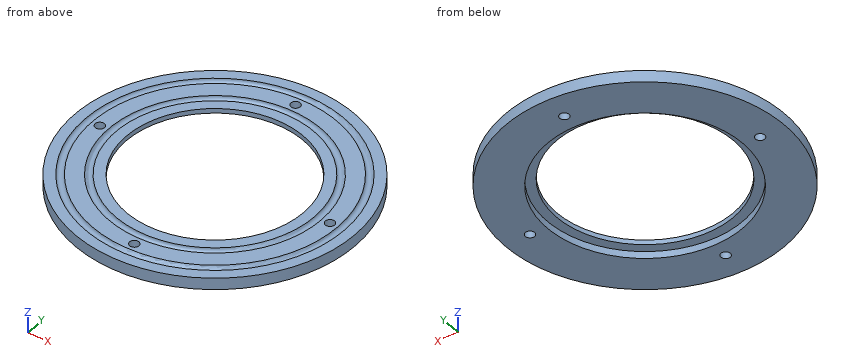
```python
from build123d import *

# Parameters (mm, degrees)
SKETCH4_R          = 2
CUT_EXTRUDE1_DEPTH = 10
SKETCH5_R          = 42
CUT_EXTRUDE2_DEPTH = 3


with BuildPart() as part:
    # Sketch3 → Revolve1 (revolve)
    with BuildSketch(Plane(origin=(0, 0, 0), x_dir=(1, 0, 0), z_dir=(0, 1, 0))):
        with BuildLine():
            Line((60, 0), (60, 5))
            Line((60, 5), (38, 5))
            Line((38, 5), (38, 0))
            Line((38, 0), (42.5, 0))
            ThreePointArc((42.5, 0), (44, 1.5), (45.5, 0))
            Line((45.5, 0), (52.5, 0))
            ThreePointArc((52.5, 0), (54, 1.5), (55.5, 0))
            Line((55.5, 0), (60, 0))
        make_face()
    revolve(axis=Axis((0, 0, 0), (0, 0, -1)))

    # Sketch4 → Cut-Extrude1 (cut)
    with BuildSketch(Plane.XY):
        with Locations((49, 0)):
            Circle(SKETCH4_R)
        with Locations((-49, 0)):
            Circle(SKETCH4_R)
        with Locations((0, 49)):
            Circle(SKETCH4_R)
        with Locations((0, -49)):
            Circle(SKETCH4_R)
    extrude(amount=-CUT_EXTRUDE1_DEPTH, mode=Mode.SUBTRACT)

    # Sketch5 → Cut-Extrude2 (cut)
    with BuildSketch(Plane(origin=(0, 0, -5), x_dir=(-1, 0, 0), z_dir=(0, 0, -1))):
        Circle(SKETCH5_R)
    extrude(amount=-CUT_EXTRUDE2_DEPTH, mode=Mode.SUBTRACT)


solid = part.part
```
Here's how the part is built. I have some questions about the finished solid (model axes, mm). Coordinates: 2 decimals unless noted, no trailing zeros. Loops run counter-clockwise (first coordinate to the right, second up) from the corner with the lowest first, then second, coordinate; pieces in that order, holes last. Notation, with made-up numbers: (66, 46.5) -> (71, 46.5) arc R10 cw to (71, 63.5) -> close; hole circle Ø7 at (-35, -12). An arc over 180 degrees is marked (long way). Return JSON: item names as keys, results as strings.
1) I need wall thicknesses on line 1 (Y direction, x = 0, z = -2.6); line 2 (Y direction, x = -24.5, z = -0.55); line 3 (Y direction, x = -1, z = -3.1). Which ranges of each line are inside material? Lowest first, please. Write a range as from..to.
Results below:
{"line 1": "-60..-51, -47..-42, 42..47, 51..60", "line 2": "-54.77..-49.68, -46.55..-38.22, -34.86..-29.05, 29.05..34.86, 38.22..46.55, 49.68..54.77", "line 3": "-59.99..-50.73, -47.27..-41.99, 41.99..47.27, 50.73..59.99"}
2) If we section it at C-C, the plane z = -3.35: Write out the boundary of the cut face in (x, y), then the cut area to 3 significant figures.
Results below:
{"outline": "circle Ø120 at (0, 0); hole circle Ø4 at (-49, 0); hole circle Ø84 at (0, 0); hole circle Ø4 at (0, -49); hole circle Ø4 at (0, 49); hole circle Ø4 at (49, 0)", "area": "5,720 mm²"}
3) If we section it at A-A, the plane x = 0: Write out the boundary of the cut face in (y, z), then the cut area to 3 significant figures.
Results below:
{"outline": "(-60, -5) -> (-51, -5) -> (-51, 0) -> (-52.5, 0) arc R1.5 cw to (-55.5, 0) -> (-60, 0) -> close; (-47, -5) -> (-42, -5) -> (-42, -2) -> (-38, -2) -> (-38, 0) -> (-42.5, 0) arc R1.5 cw to (-45.5, 0) -> (-47, 0) -> close; (38, -2) -> (42, -2) -> (42, -5) -> (47, -5) -> (47, 0) -> (45.5, 0) arc R1.5 cw to (42.5, 0) -> (38, 0) -> close; (51, -5) -> (60, -5) -> (60, 0) -> (55.5, 0) arc R1.5 cw to (52.5, 0) -> (51, 0) -> close", "area": "142 mm²"}
4) Will these pins go through, and if not, where does the flat tip stop? pin 1 (6 mm diameter, centred on x = 36, y = -8.5, fed in from -Z); pin 2 (2 mm diameter, centred on y = 20.5, z = -4.5, fed in from +X); pin 3 (2 mm diameter, centred on y = -7.5, z = -2.5, fed in from -X); pin 4 (3.5 mm diameter, centred on x = 0, y = 49, fed in from -Z).
Results below:
{"pin 1": "z = -2", "pin 2": "x = 56.74", "pin 3": "x = -59.65", "pin 4": "through"}
